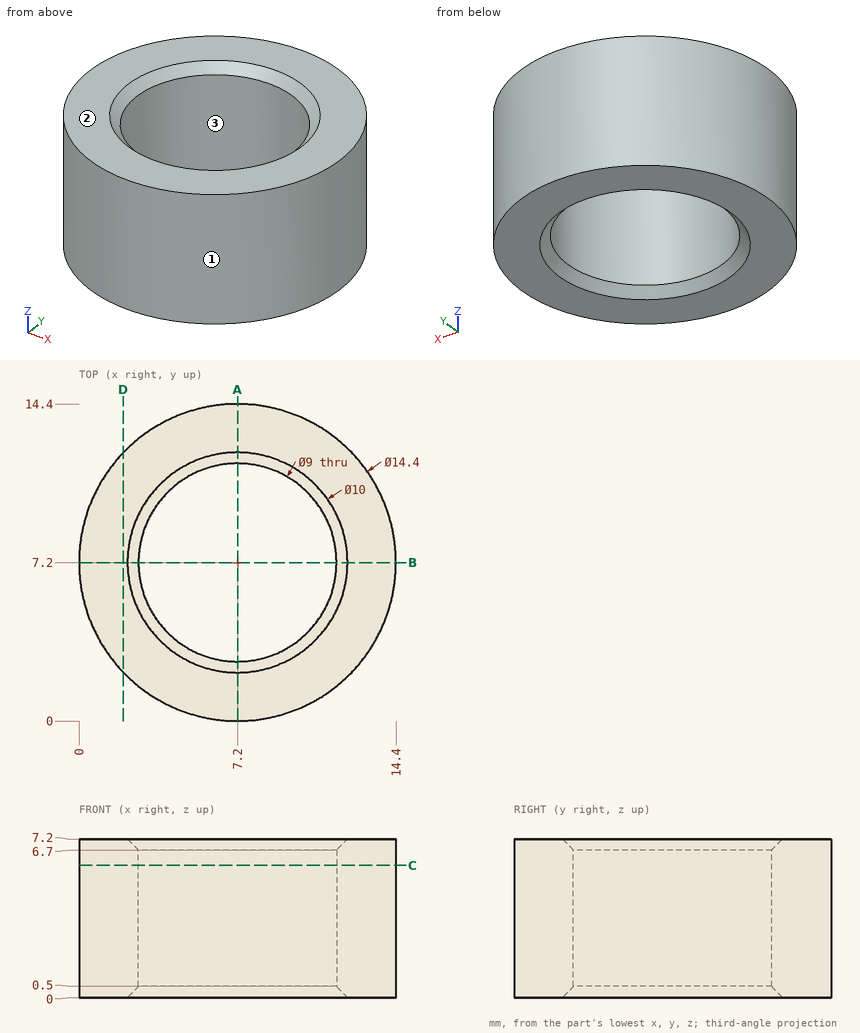
Geometry: see drawing. Coordinates: mm, zero at the bounding-box minimum. Give positions to 0.01 mm unless a question says otherwise; leave off trailing zeros. Write each loop counter-clockwise with the first axis right and the second up, starting at its lowest first coordinate (ties: lowest second). Pieces come first, ordered by that corner, then holes. Notation, with made-up numbers: (55, 25.5) - (81, 25.5) arc R32 ccw to (81, 60.5) - close; hole circle Ø8 at (44.25, -20). An arc over 180 degrees is marked (long way). Return JSON: item names as keys, results as strings. Group by question number.
1) Section D-D on x = 2. Return the cut outline in (y, z).
2) Line query: line 1 (Y direction, x = 7.2, z = 2); line 2 (X direction, y = 7.75, z = 1.5); line 3 (X direction, y = 11, z = 2.5). Output: solid intervals per line, ascending.
3) Section C-C on z = 6. Return the cut outline in (x, y).
4) Section A-A on x = 7.2. Return the cut outline in (y, z), plus the area to 3 significant figures.
5) First-contact query: P1, Ø5.5, axis at x = 7.2, y = 7.2, coming from the -Z side. Flat tip, straight axial feed; report the tip coordinate or a pass-through.
6) Mould query, pull axis Y, two halves, no side actions, for the marked faces 1, 2 and 3. Classes: released by +Y, released by -Y, zero draft, split by the parting line, or undercut.
Filled in:
{
 "1": {"outline": "(2.22, 0) - (12.18, 0) - (12.18, 7.2) - (2.22, 7.2) - close"},
 "2": {"line 1": "y = 0 to 2.7, 11.7 to 14.4", "line 2": "x = 0.02 to 2.73, 11.67 to 14.38", "line 3": "x = 1.08 to 4.79, 9.61 to 13.32"},
 "3": {"outline": "circle Ø14.4 at (7.2, 7.2); hole circle Ø9 at (7.2, 7.2)"},
 "4": {"outline": "(0, 0) - (2.2, 0) - (2.7, 0.5) - (2.7, 6.7) - (2.2, 7.2) - (0, 7.2) - close; (11.7, 0.5) - (12.2, 0) - (14.4, 0) - (14.4, 7.2) - (12.2, 7.2) - (11.7, 6.7) - close", "area": "38.4 mm^2"},
 "5": {"P1": "passes through"},
 "6": {"face 1": "split by the parting line", "face 2": "zero draft", "face 3": "undercut"}
}
